Could you check a few things on this model? Use its own coordinates, in mm. A direction names the side the tool comes from. Coordinates: 2 decimals unless noted, no trailing zeros. Order: outer loops, then holes, each group sorted by start corner. A loop starts at its lowest first (then second) coordinate and runs counter-clockwise, first axis right, second up. Notation, with made-up numbers: M 43.5,-26.5 L 99.5,-26.5 A19 ccw 99.5,4.5 Z; hole C 15.5,73 d10. An arc over 180 degrees is marked long. One line per question, with ' | ' between items. Start each with the question number.
Autodesk Inventor part; units mm, degrees
ref_plane "YZ Plane" through (0, 0, 0) normal (1, 0, 0) x (0, 1, 0)
ref_plane "XZ Plane" through (0, 0, 0) normal (0, 1, 0) x (-1, 0, 0)
ref_plane "XY Plane" through (0, 0, 0) normal (0, 0, 1) x (1, 0, 0)
sketch "Sketch1" plane through (0, 0, 0) normal (0, 0, 1) x (1, 0, 0)
  line L0 (25, -7) -> (50, -7)
  line L1 (50, 45.5218) -> (50, -7)
  line L2 (50, 45.5218) -> (11.4158, 45.5218)
  line L3 (11.4158, 45.5218) -> (11.4158, 48.5218)
  line L4 (11.4158, 48.5218) -> (-11.4158, 48.5218)
  line L5 (-11.4158, 48.5218) -> (-11.4158, 45.5218)
  line L6 (-11.4158, 45.5218) -> (-50, 45.5218)
  line L7 (-50, 45.5218) -> (-50, -7)
  line L8 (-50, -7) -> (-25, -7)
  line L9 (-25, -7) -> (-25, -24)
  line L10 (-25, -24) -> (-32.4371, -24)
  line L11 (-32.4371, -24) -> (-32.4371, -28)
  line L12 (-32.4371, -28) -> (-25, -28)
  line L13 (-25, -28) -> (-25, -35)
  line L14 (-25, -35) -> (25, -35)
  line L15 (25, -35) -> (25, -28)
  line L16 (25, -28) -> (30.7079, -28)
  line L17 (30.7079, -28) -> (30.7079, -24)
  line L18 (30.7079, -24) -> (25, -24)
  line L19 (25, -24) -> (25, -7)
  circle A0 centre (-11.4158, 26.1989) radius 1.6
  circle A1 centre (20.9961, 37.6953) radius 1.6
  circle A2 centre (-20.9961, 37.6953) radius 1.6
  circle A3 centre (11.4158, 26.1989) radius 1.6
  line L20 (15.6, -21.3595) -> (2, -21.3595)
  line L21 (-2, -21.3109) -> (-15.6, -21.3109)
  line L22 (-2.4, -19.4751) -> (-15.6, -19.4751)
  line L23 (2.4, -19.5236) -> (15.6, -19.5236)
  line L24 (50, -7) -> (-50, -7)
  line L25 (-50, -7) -> (-50, 20.7683)
  line L26 (-50, 20.7683) -> (50, 20.7683)
  line L27 (50, 20.7683) -> (50, -7)
  point P0 (0, 0)
extrude "Extrusion1" add sketch "Sketch1" along normal blind 13 contours L24 L8 L7 L26 L1 L0
sketch "Sketch2" plane through (0, 0, 13) normal (0, 0, 1) x (1, 0, 0)
  line L0 (25, -7) -> (50, -7)
  line L1 (50, 45.5218) -> (50, -7)
  line L2 (50, 45.5218) -> (11.4158, 45.5218)
  line L3 (11.4158, 45.5218) -> (11.4158, 48.5218)
  line L4 (11.4158, 48.5218) -> (-11.4158, 48.5218)
  line L5 (-11.4158, 48.5218) -> (-11.4158, 45.5218)
  line L6 (-11.4158, 45.5218) -> (-50, 45.5218)
  line L7 (-50, 45.5218) -> (-50, -7)
  line L8 (-50, -7) -> (-25, -7)
  line L9 (-25, -7) -> (-25, -24)
  line L10 (-25, -24) -> (-32.4371, -24)
  line L11 (-32.4371, -24) -> (-32.4371, -28)
  line L12 (-32.4371, -28) -> (-25, -28)
  line L13 (-25, -28) -> (-25, -35)
  line L14 (-25, -35) -> (25, -35)
  line L15 (25, -35) -> (25, -28)
  line L16 (25, -28) -> (30.7079, -28)
  line L17 (30.7079, -28) -> (30.7079, -24)
  line L18 (30.7079, -24) -> (25, -24)
  line L19 (25, -24) -> (25, -7)
  circle A0 centre (-11.4158, 26.1989) radius 1.6
  circle A1 centre (20.9961, 37.6953) radius 1.6
  circle A2 centre (-20.9961, 37.6953) radius 1.6
  circle A3 centre (11.4158, 26.1989) radius 1.6
  line L20 (50, 20.7683) -> (-50, 20.7683)
  line L21 (-50, 20.7683) -> (50, 20.7683)
  line L22 (50, 20.7683) -> (50, -35)
  line L23 (50, -35) -> (-50, -35)
  line L24 (-50, -35) -> (-50, 20.7683)
  point P0 (0, 0)
extrude "Extrusion2" add sketch "Sketch2" along normal blind 20 contours L19 L18 L17 L16 L15 L14 L13 L12 L11 L10 L9 L8 L7 L20 L1 L0 | L0 L22 L23 L15 L16 L17 L18 L19 | L8 L9 L10 L11 L12 L13 L23 L24
(1) If I drill on line 1 along Z through (x, y) = (-24.5, -19.5); line 2 along Y through (x, z) = (-41, 12.5), over which ranges is the centre line in solid material (lowest first)? Write a range as from..to.
(2) On a 3-axis mill with a long thin cutter (end or side, diameter ignored), from which of +Z, -Z, +X, -X, +Y, -Y can I reach the whole of each face in a straight line? I mean faces 1 (the flat face through (-1, 7, 0)), 2 (the flat face through (-1, -21, 13)). Say none if no direction works.
(3) Imagine slicing it at C-C, the plane z = 6. Write out the boundary of the cut face in (x, y), plus the area to 3 significant figures.
(4) Imagine slicing it at A-A, the plane x = -14. Write out the boundary of the cut face in (y, z), plus the area to 3 significant figures.
(5) Imagine slicing it at B-B, the plane y = -14. Write out the boundary of the cut face in (x, z).
(6) For P1, Ø6, axis at x = -2, y = -20.5, coming from the -Z side; P2, Ø14.5, axis at x = 22.5, z = 4.5, coming from the -Y side, each with a flat end and sliding along its axis, tell me the tip position at first contact or that it passes through.
Answers:
1) line 1: 13..33 | line 2: -7..20.77
2) face 1: -Z, +X, -X, +Y, -Y | face 2: -Z, +X, -X, -Y
3) outline: M -50,-7 L 50,-7 L 50,20.77 L -50,20.77 Z | area: 2,780 mm²
4) outline: M -35,13 L -7,13 L -7,0 L 20.77,0 L 20.77,33 L -35,33 Z | area: 1,480 mm²
5) outline: M -50,13 L 50,13 L 50,33 L -50,33 Z
6) P1: z = 13 | P2: y = -7
